Part print with two shaded views. Sizes in mm from the minimum x, y, z corner. A direction names the side the tool comes from. Round coordinates to 2 decimals unless told otherwise and drop trailing zeros. Order: outer loops, then holes, each group sorted by start corner. A loop starts at its lowest first (then second) coordinate and runs counter-clockwise, first axis right, second up. Notation, with made-up numbers: (45, -39) -> (60, -39) arc R19 ccw to (60, -14) -> close; hole circle Ø9 at (49, 87.5). An arc over 180 degrees is marked (long way). Answer as a JSON object with one key per item and string values.
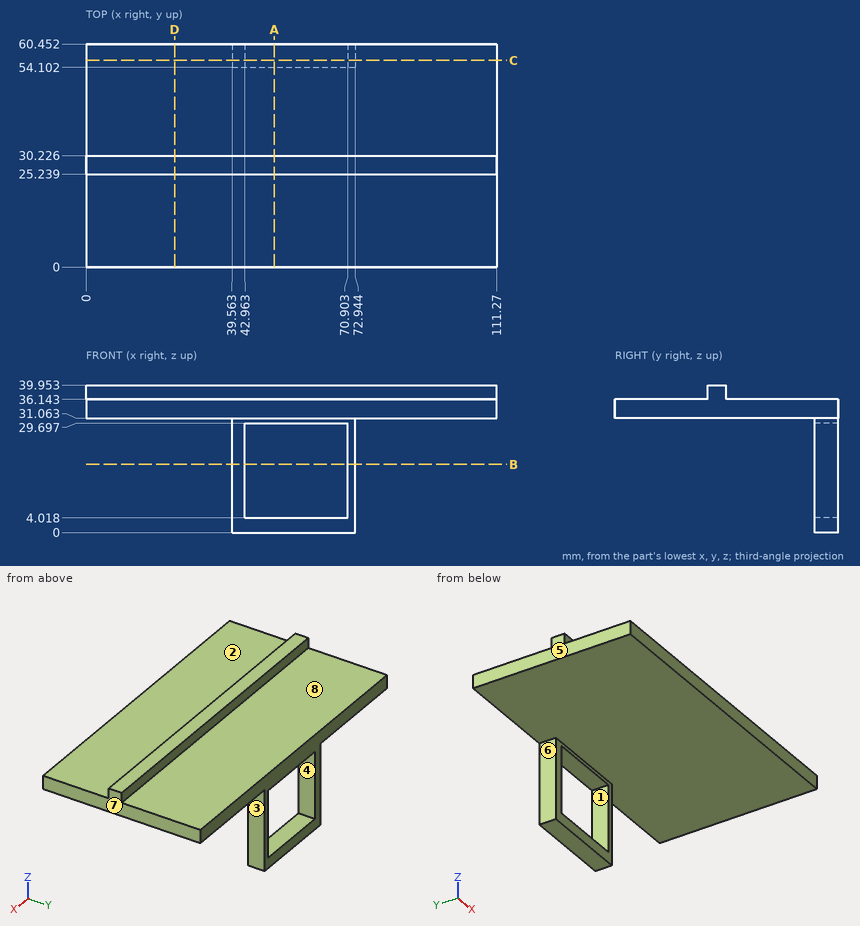
1) Which spindle directions (+Z, -Z, +X, -X, +Y, -Y) get a long thin tool onto all of the face, cutting with end or side? Do the marked faces 4, 5, 6, 7 and 8. Say none if no direction does.
Checked values:
{"face 4": "+Y, -Y", "face 5": "+Z, -Z, -X, +Y, -Y", "face 6": "-Z, -X, +Y, -Y", "face 7": "+Z, -Z, +X, +Y, -Y", "face 8": "+Z, +X, -X, +Y"}
2) Probe L1, parallel to X at y = 57.5, z = 5; L2, parallel to Z at x = 72, y = 51; L3, parallel to Y at x = 48.5, z = 3. List the from-to ranges inside material, lowest first. Write a range as from..to.
Checked values:
{"L1": "x = 39.56..42.96, 70.9..72.94", "L2": "z = 31.06..36.14", "L3": "y = 54.1..60.45"}
3) Cut at C-C, the plane y = 56. Give the cut face in (x, z).
Checked values:
{"outline": "(0, 31.06) -> (39.56, 31.06) -> (39.56, 0) -> (72.94, 0) -> (72.94, 31.06) -> (111.27, 31.06) -> (111.27, 36.14) -> (0, 36.14) -> close; hole (42.96, 4.02) -> (70.9, 4.02) -> (70.9, 29.7) -> (42.96, 29.7) -> close"}
4) Pull direction Z, two halves, no side cores. Call the marked faces 1, 2 and 3: pulls with the +Z half, pulls with the -Z half, needs draft (parallel to the pull), parting line crosses it, or undercut.
Checked values:
{"face 1": "undercut", "face 2": "pulls with the +Z half", "face 3": "needs draft"}
5) Cut at A-A, the plane x = 51. Give the cut face in (y, z) (1 decimal), plus the area to 3 significant figures.
Checked values:
{"outline": "(0, 31.1) -> (54.1, 31.1) -> (54.1, 29.7) -> (60.5, 29.7) -> (60.5, 36.1) -> (30.2, 36.1) -> (30.2, 40) -> (25.2, 40) -> (25.2, 36.1) -> (0, 36.1) -> close; (54.1, 0) -> (60.5, 0) -> (60.5, 4) -> (54.1, 4) -> close", "area": "360 mm²"}
6) Flat gauge pins, fed straight in: pin 1 Ø5 at (y, z) = (57.5, 16) entering from +X; pin 2 Ø1.1 at (x, z) = (58, 37.5) entering from -Y; pin 3 Ø3 at (y, z) = (56, 21.5) entering from -X. Where does each tip first touch, or does it go through?
Checked values:
{"pin 1": "stops at x = 72.94", "pin 2": "stops at y = 25.24", "pin 3": "stops at x = 39.56"}
7) Cut at B-B, the plane z = 18.5. Give the cut face in (x, y).
Checked values:
{"outline": "(39.56, 54.1) -> (42.96, 54.1) -> (42.96, 60.45) -> (39.56, 60.45) -> close; (70.9, 54.1) -> (72.94, 54.1) -> (72.94, 60.45) -> (70.9, 60.45) -> close"}
8) Cut at D-D, the plane x = 24. Give the cut face in (y, z) (1 decimal), plus the area to 3 significant figures.
Checked values:
{"outline": "(0, 31.1) -> (60.5, 31.1) -> (60.5, 36.1) -> (30.2, 36.1) -> (30.2, 40) -> (25.2, 40) -> (25.2, 36.1) -> (0, 36.1) -> close", "area": "326 mm²"}
